Here's how the part is built. I have some questions about the finished solid (model axes, mm). Give positions to 0.01 mm unless a question says otherwise; leave off trailing zeros. Write each loop counter-clockwise with the first axis right and the second up, starting at its lowest first coordinate (ties: lowest second). Pieces come first, ordered by that corner, then holes. Notation, with made-up numbers: (8.5, 52) - (15.5, 52) arc R19 ccw to (15.5, 87) - close; hole circle Ø10 at (74.25, -22.5). An arc over 180 degrees is marked (long way). Use a Markdown table: item, result.
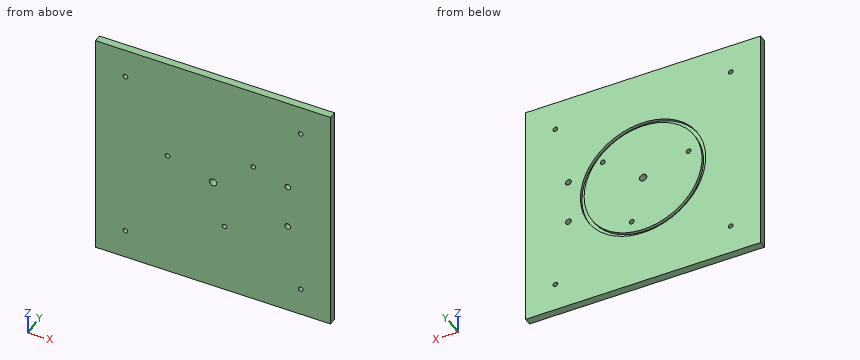
```python
from build123d import *

# Parameters (mm, degrees)
SKETCH1_W                  = 200
SKETCH1_H                  = 200
BOSS_EXTRUDE1_DEPTH        = 6.35
SKETCH2_R                  = 3.175
CUT_EXTRUDE1_DEPTH         = 7.35
SKETCH3_R                  = 2.4892
CUT_EXTRUDE2_DEPTH         = 7.35
SKETCH4_R                  = 53.34
SKETCH4_R_2                = 50.165
CUT_EXTRUDE3_DEPTH         = 2.54
F_10_32_TAPPED_HOLE1_D     = 4.0386
F_10_32_TAPPED_HOLE1_DEPTH = 13.716
F_10_32_TAPPED_HOLE1_TIP   = 1.213317848
SKETCH9_R                  = 2.02
SKETCH9_R_2                = 2.032
CUT_EXTRUDE4_DEPTH         = 7.35


with BuildPart() as part:
    # Sketch1 → Boss-Extrude1 (new body)
    with BuildSketch(Plane(origin=(0, 0, 0), x_dir=(1, 0, 0), z_dir=(0, 1, 0))):
        Rectangle(SKETCH1_W, SKETCH1_H)
    extrude(amount=BOSS_EXTRUDE1_DEPTH)

    # Sketch2 → Cut-Extrude1 (cut, through all)
    with BuildSketch(Plane(origin=(0, 6.35, 0), x_dir=(1, 0, 0), z_dir=(0, 1, 0))):
        Circle(SKETCH2_R)
    extrude(amount=-CUT_EXTRUDE1_DEPTH, mode=Mode.SUBTRACT)

    # Sketch3 → Cut-Extrude2 (cut, through all)
    with BuildSketch(Plane(origin=(0, 6.35, 0), x_dir=(1, 0, 0), z_dir=(0, 1, 0))):
        with Locations((63.5, -19.05)):
            Circle(SKETCH3_R)
        with Locations((63.5, 19.05)):
            Circle(SKETCH3_R)
    extrude(amount=-CUT_EXTRUDE2_DEPTH, mode=Mode.SUBTRACT)

    # Sketch4 → Cut-Extrude3 (cut)
    with BuildSketch(Plane(origin=(0, 6.35, 0), x_dir=(1, 0, 0), z_dir=(0, 1, 0))):
        Circle(SKETCH4_R)
        Circle(SKETCH4_R_2, mode=Mode.SUBTRACT)
    extrude(amount=-CUT_EXTRUDE3_DEPTH, mode=Mode.SUBTRACT)

    # #10-32 Tapped Hole1
    with Locations(Plane(origin=(0, 6.35, 0), x_dir=(1, 0, 0), z_dir=(0, 1, 0))):
        with Locations((9.693302756, 39.140054777), (-38.74293312, -11.175380955), (34.225642894, -27.683137416)):
            Hole(F_10_32_TAPPED_HOLE1_D / 2, depth=F_10_32_TAPPED_HOLE1_DEPTH)
            with Locations((0, 0, -(F_10_32_TAPPED_HOLE1_DEPTH + F_10_32_TAPPED_HOLE1_TIP / 2))):  # 118° drill point
                Cone(0, F_10_32_TAPPED_HOLE1_D / 2, F_10_32_TAPPED_HOLE1_TIP, mode=Mode.SUBTRACT)

    # Sketch9 → Cut-Extrude4 (cut, through all)
    with BuildSketch(Plane(origin=(0, 6.35, 0), x_dir=(1, 0, 0), z_dir=(0, 1, 0))):
        with Locations((-74.6, 74.6)):
            Circle(SKETCH9_R)
        with Locations((74.6, 75.660597777)):
            Circle(SKETCH9_R)
        with Locations((74.6, -74.6)):
            Circle(SKETCH9_R)
        with Locations((-74.6, -74.6)):
            Circle(SKETCH9_R_2)
    extrude(amount=-CUT_EXTRUDE4_DEPTH, mode=Mode.SUBTRACT)


solid = part.part
```
Item 1: If we section it at A-A, the plane x = 63.5: Write out the boundary of the cut face in (y, z), plus the area to 3 significant figures.
Values:
| item | result |
|---|---|
| outline | (0, -100) - (6.35, -100) - (6.35, -21.54) - (0, -21.54) - close; (0, -16.56) - (6.35, -16.56) - (6.35, 16.56) - (0, 16.56) - close; (0, 21.54) - (6.35, 21.54) - (6.35, 100) - (0, 100) - close |
| area | 1,210 mm2 |
Item 2: I need wall thicknesses on line 1 along X through (y, z) = (4.6, 0) (3 decimals); line 2 along Z through (x, y) = (73, 0.75). Which ranges of each line are inside material? Lowest first, please. Write a range as [from, to].
Values:
| item | result |
|---|---|
| line 1 | x = [-100, -53.34], [-50.165, -3.175], [3.175, 50.165], [53.34, 100] |
| line 2 | z = [-100, -76.89], [-74.43, 73.37], [75.83, 100] |
Item 3: If we section it at B-B, the plane z = 19.05: Write out the boundary of the cut face in (x, y).
Values:
| item | result |
|---|---|
| outline | (-100, 0) - (61.01, 0) - (61.01, 6.35) - (49.82, 6.35) - (49.82, 3.81) - (46.41, 3.81) - (46.41, 6.35) - (-46.41, 6.35) - (-46.41, 3.81) - (-49.82, 3.81) - (-49.82, 6.35) - (-100, 6.35) - close; (65.99, 0) - (100, 0) - (100, 6.35) - (65.99, 6.35) - close |
